from build123d import *

# Parameters (mm, degrees)
TORUS_R        = 0.6
CYLINDER_R     = 7
CYLINDER_DEPTH = 12
FILLET001_R    = 0.5


with BuildPart() as torus:
    # Torus → Torus (revolve)
    with BuildSketch(Plane(origin=(10, 10, 12), x_dir=(1, 0, 0), z_dir=(0, -1, 0))):
        with Locations((5, 0)):
            Circle(TORUS_R)
    revolve(axis=Axis((10, 10, 12), (0, 0, 1)))


with BuildPart() as cut001:
    # Cylinder → Cylinder (new body)
    with BuildSketch(Plane(origin=(10, 10, 0), x_dir=(1, 0, 0), z_dir=(0, 0, 1))):
        Circle(CYLINDER_R)
    extrude(amount=CYLINDER_DEPTH)

    # Fillet001
    fillet001_edges = [cut001.edges().sort_by_distance(p)[0] for p in [
        (3, 10, 12),
    ]]
    fillet(fillet001_edges, radius=FILLET001_R)

    # Cut001: cut Torus
    add(torus.part, mode=Mode.SUBTRACT)


solid = cut001.part
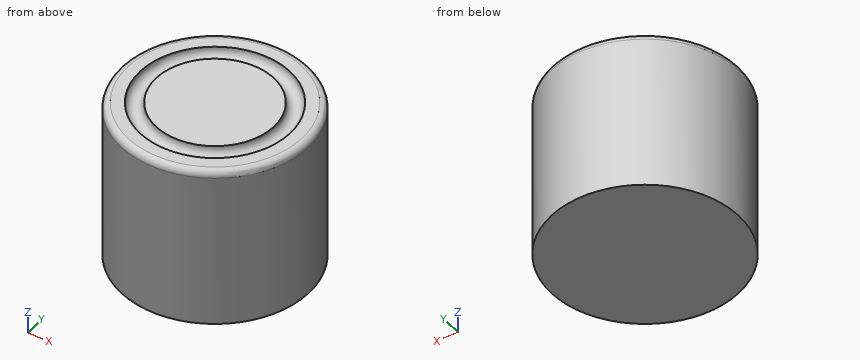
Build history of the part. All positions in model axes, mm. Round coordinates to 2 decimals unless told otherwise and drop trailing zeros. Write each loop counter-clockwise with the first axis right and the second up, starting at its lowest first coordinate (ties: lowest second). Pieces come first, ordered by that corner, then holes. Notation, with made-up numbers: M 13.25,89.5 L 56.25,89.5 A23 ccw 56.25,109.5 Z; hole C 64,37 d1. An arc over 180 degrees is marked long. Use CSV: the item, a comma, the result in double quotes.
1. Wall check: probe 1 along Y at (x, z) = (5.25, 11.75); probe 2 along Y at (x, z) = (10.75, 0.5); probe 3 along Y at (x, z) = (15, 3.25). Give the ranges that are in metal, low to high. Write a range as from..to.
Reply:
probe 1,"y = 4.95..7.14, 12.86..15.05"
probe 2,"y = 3.04..16.96"
probe 3,"y = 5.1..14.9"
2. Flat gauge pins, fed straight in: pin 1 (4 mm diameter, centred on x = 7, z = 3, fed in from +Y); pin 2 (4 mm diameter, centred on x = 12, z = 10, fed in from +Y); pin 3 (2 mm diameter, centred on y = 6.5, z = 5.5, fed in from -X). Where does each tip first touch, or does it go through?
Reply:
pin 1,"stops at y = 16.93"
pin 2,"stops at y = 17"
pin 3,"stops at x = 3.46"
3. Saw through at A-A (z = 7.5). Give the cut face in (x, y), plus the area to 3 significant figures.
Reply:
outline,"C 10,10 d14"
area,"154 mm²"
